Here's how the part is built. I have some questions about the finished solid (model axes, mm). Give positions to 0.01 mm unless a question says otherwise; leave off trailing zeros. Write each loop counter-clockwise with the first axis right and the second up, starting at its lowest first coordinate (ties: lowest second). Pieces come first, ordered by that corner, then holes. Notation, with made-up numbers: (55, -17.75) - (61, -17.75) arc R13 cw to (61, 6.25) - close; hole circle Ø3 at (2.5, 54). An arc over 180 degrees is marked (long way). Use one line per item in the form item = value. Start each with the question number.
from build123d import *

# Parameters (mm, degrees)
F0_W     = 13.97
F0_H     = 5.08
F1_DEPTH = 1.524
F2_R     = 1.27
F3_DEPTH = 25.4
F4_R     = 2.53999


# Not quite as in the source:
# - a fillet or chamfer is up to 0.001 mm smaller than in the source, because OpenCascade refuses the exact size


with BuildPart() as f1:
    # F0 (on Top) → F1 (new body)
    with BuildSketch(Plane.XY):
        with Locations((6.985, 2.54)):
            Rectangle(F0_W, F0_H)
    extrude(amount=F1_DEPTH)

    # F2 (on face) → F3 (cut)
    with BuildSketch(Plane.XY.offset(1.524)):
        with Locations((3.175, 2.54)):
            Circle(F2_R)
    extrude(amount=-F3_DEPTH, mode=Mode.SUBTRACT)

    # F4 (radius 2.54 in the source; OpenCascade refuses exactly that, so slightly less here)
    f4_edges = [f1.edges().sort_by_distance(p)[0] for p in [
        (0, 0, 0.762),
        (0, 5.08, 0.762),
    ]]
    fillet(f4_edges, radius=F4_R)


solid = f1.part
1. Please list where these lines run through material, in increasing order: line 1 (Y direction, x = 2.5, z = 0.6); line 2 (X direction, y = 2.85, z = 0.5); line 3 (X direction, y = 2, z = 1).
2. I want a section at C-C, the plane y = 2.4. List the corners of the cut face in (x, z) for me, then the cut area to 3 significant figures.
3. I want a section at D-D, the plane y = 0.85. List the corners of the cut face in (x, z) for me, then the cut area to 3 significant figures.
4. I want a section at A-A, the plane x = 3.5. List the corners of the cut face in (y, z) for me.
Result sheet:
q1.line_1 = 0 to 1.46, 3.62 to 5.08
q1.line_2 = 0.02 to 1.94, 4.41 to 13.97
q1.line_3 = 0.06 to 2.03, 4.32 to 13.97
q2.outline = (0, 0) - (1.91, 0) - (1.91, 1.52) - (0, 1.52) - close; (4.44, 0) - (13.97, 0) - (13.97, 1.52) - (4.44, 1.52) - close
q2.area = 17.4 mm2
q3.outline = (0.64, 0) - (13.97, 0) - (13.97, 1.52) - (0.64, 1.52) - close
q3.area = 20.3 mm2
q4.outline = (0, 0) - (1.31, 0) - (1.31, 1.52) - (0, 1.52) - close; (3.77, 0) - (5.08, 0) - (5.08, 1.52) - (3.77, 1.52) - close
